from build123d import *

# Parameters (mm, degrees)
F2_R    = 4.5
F3_SIZE = 1.2
F4_R    = 0.2


with BuildPart() as f1:
    # F0 (on Front) → F1 (revolve)
    with BuildSketch(Plane.XZ):
        Polygon((-2.4, -40.570669), (-5, -40.570669), (-5, -146.320669), (0, -146.320669), (0, -28.570669), (-2.4, -28.570669), align=None)
    revolve(axis=Axis((0, 0, -136.627736), (0, 0, -1)))

    # F2
    f2_edges = [f1.edges().sort_by_distance(p)[0] for p in [
        (5, 0, -146.320669),
    ]]
    fillet(f2_edges, radius=F2_R)

    # F3
    f3_edges = [f1.edges().sort_by_distance(p)[0] for p in [
        (2.4, 0, -28.570669),
    ]]
    chamfer(f3_edges, length=F3_SIZE)

    # F4
    f4_edges = [f1.edges().sort_by_distance(p)[0] for p in [
        (2.4, 0, -40.570669),
    ]]
    fillet(f4_edges, radius=F4_R)


solid = f1.part
Verification items for the finished model (mm, model axes). A direction names the side the tool comes from. Round coordinates to 2 decimals unless told otherwise and drop trailing zeros. Order: outer loops, then holes, each group sorted by start corner. A loop starts at its lowest first (then second) coordinate and runs counter-clockwise, first axis right, second up. Notation, with made-up numbers: (70, -3) -> (99, -3) arc R36 cw to (99, 31) -> close; hole circle Ø11 at (42, 28.5). An arc over 180 degrees is marked (long way). Put each result on its own line as item: value.
1) Material ranges on line 1 (X direction, y = 0.25, z = -140); line 2 (X direction, y = 2, z = -124), recorded low to high.
Final values:
line 1: x = -4.99 to 4.99
line 2: x = -4.58 to 4.58
2) Set-up check for faces 1 (the flat face through (0, 0, -28.571)), 2 (the cylindrical face through (-1.29, 2.024, -35.145)): record each of +Z, -Z, +X, -X, +Y, -Y from which the full face is reachable in a straight line by a thin tool's end or side.
Final values:
face 1: +Z, +X, -X, +Y, -Y
face 2: +Z
3) Section check A-A (z = -42.5). Record the cut outline in (x, y), then the cut area to 3 significant figures.
Final values:
outline: circle Ø10 at (0, 0)
area: 78.5 mm^2
4) Depth check by flat-ended pin: pin 1 (1 mm diameter, centred on x = -0.5, y = -3.5, fed in from +Z); pin 2 (2 mm diameter, centred on x = 0.5, y = -2.5, fed in from +Z). Enter the tip coordinate at first touch or a pass-through.
Final values:
pin 1: stops at z = -40.57
pin 2: stops at z = -28.92
